Solid Edge part; units mm, degrees
sketch "Sketch1" plane through (0, 0, 0) normal (0, 0, 1) x (1, 0, 0)
  line L0 (12.5075, 35.7826) -> (12.5075, 18.7826)
  line L1 (12.5075, 18.7826) -> (30.5075, 18.7826)
  line L2 (30.5075, 18.7826) -> (46.9075, -0.2273)
  line L3 (46.9075, -0.2273) -> (46.9075, -32.2273)
  line L4 (46.9075, -32.2273) -> (-27.0925, -32.2273)
  line L5 (-27.0925, -32.2273) -> (-27.0925, -0.7273)
  line L6 (-27.0925, -0.7273) -> (-60.0925, -0.7273)
  line L7 (-60.0925, -0.7273) -> (-60.0925, 29.7727)
  line L8 (-60.0925, 29.7727) -> (-27.0925, 29.7727)
  line L9 (-27.0925, 29.7727) -> (12.5075, 35.7826)
  dimension "D1" = 46.9075
  dimension "D2" = 46.9075
  dimension "D3" = 27.0925
  dimension "D4" = 27.0925
  dimension "D5" = 60.0925
  dimension "D6" = 60.0925
  dimension "D7" = 12.5075
  dimension "D8" = 12.5075
extrude "Ajout_matière_1" add sketch "Sketch1" along normal blind 12
sketch "Sketch2" plane through (-11.8425, 1.7776, 12) normal (0, 0, 1) x (1, 0, 0)
  line L0 (-45.25, 24.995) -> (-45.25, 0.495)
  line L1 (-45.25, 0.495) -> (18.1748, 0.495)
  line L2 (44.4511, 0.495) -> (43.1748, 0.495)
  line L3 (39.9995, 14.005) -> (44.4511, 0.495)
  line L4 (21.35, 14.005) -> (39.9995, 14.005)
  line L5 (21.35, 29.6711) -> (21.35, 14.005)
  line L6 (-12.3173, 24.995) -> (21.35, 29.6711)
  line L7 (-45.25, 24.995) -> (-12.3173, 24.995)
  arc A0 (18.1748, 0.495) -> (43.1748, 0.495) centre (30.6748, 0.495) ccw
extrude "Enlèvement_matière_1" cut sketch "Sketch2" against normal blind 11
sketch "Sketch3" plane through (-12.2419, 10.6107, 1) normal (0, 0, 1) x (1, 0, 0)
  circle A0 centre (31.0742, -8.338) radius 1.2899
extrude "Cutout1" cut sketch "Sketch3" along normal through all and the other way through all
sketch "Sketch4" plane through (-11.8425, 1.7776, 0) normal (0, 0, -1) x (0, 1, 0)
  line L0 (-34.005, 58.75) -> (-4.005, 58.75)
  line L1 (-4.005, 58.75) -> (-4.005, -15.25)
  line L2 (-4.005, -15.25) -> (-34.005, -15.25)
  line L3 (-34.005, -15.25) -> (-34.005, 15.75)
  line L4 (-25.505, 15.75) -> (-34.005, 15.75)
  line L5 (-25.505, 26.25) -> (-25.505, 15.75)
  line L6 (-34.005, 26.25) -> (-25.505, 26.25)
  line L7 (-34.005, 26.25) -> (-34.005, 58.75)
  dimension "D1" = 34.005
  dimension "D2" = 25.505
  dimension "D3" = 34.005
extrude "Enlèvement_matière_3" cut sketch "Sketch4" against normal blind 6
sketch "Sketch5" plane through (-6.5925, 1.7776, 12) normal (0, 0, 1) x (0, -1, 0)
  circle A0 centre (28.505, 49) radius 1.5
  circle A1 centre (28.505, 38) radius 1.5
  circle A2 centre (28.505, -5) radius 1.5
  line L0 (24.905, 13) -> (32.105, 13)
  line L1 (32.105, 13) -> (32.105, 6.5)
  line L2 (32.105, 6.5) -> (24.905, 6.5)
  line L3 (24.905, 6.5) -> (24.905, 13)
  dimension "D1" = 28.505
extrude "Cutout2" cut sketch "Sketch5" along normal through all and the other way through all
sketch "Sketch6" plane through (-12.2419, 14.6107, 1) normal (0, 0, 1) x (0, -1, 0)
  circle A0 centre (-8.1719, -6.8505) radius 1.5
  dimension "D1" = 8.1719
extrude "Cutout3" cut sketch "Sketch6" along normal through all and the other way through all
sketch "Sketch7" plane through (-6.5925, 1.7776, 12) normal (0, 0, 1) x (0, -1, 0)
  circle A0 centre (18.005, 46.5) radius 1.5
extrude "Cutout4" cut sketch "Sketch7" along normal through all and the other way through all
sketch "Sketch8" plane through (-6.5925, 1.7776, 12) normal (0, 0, 1) x (-1, 0, 0)
  line L0 (20.5, 2.505) -> (58.2278, 2.505)
  line L1 (58.2278, 2.505) -> (58.2278, -30.8265)
  line L2 (58.2278, -30.8265) -> (20.5, -30.8265)
  line L3 (20.5, -30.8265) -> (20.5, 2.505)
  dimension "D1" = 20.5
  dimension "D2" = 58.2278
extrude "Enlèvement_matière_7" cut sketch "Sketch8" along normal mid plane 65.5466
properties material "Nylon, usage général"
Design review of the part built by this model. Coordinates are the model's own, in mm. A direction names the side the tool comes from. Round coordinates to 2 decimals unless told otherwise and drop trailing zeros. Write each loop counter-clockwise with the first axis right and the second up, starting at its lowest first coordinate (ties: lowest second). Pieces come first, ordered by that corner, then holes. Notation, with made-up numbers: (-4, 80.25) - (33, 80.25) arc R36 cw to (33, 117.25) - close; hole circle Ø2 at (7, 14.5). An arc over 180 degrees is marked (long way). Use a Markdown table: item, result. Add a question column.
1. Clearance check with flat-ended pins moving along their axes: pin 1 (4 mm diameter, centred on x = -19.09, y = 22.78, fed in from +Z); pin 2 (1.8 mm diameter, centred on x = 11.5, z = 3, fed in from +Y); pin 3 (6 mm diameter, centred on y = 20, z = 8.5, fed in from +X); pin 4 (2.5 mm diameter, centred on x = 31.41, y = -26.73, fed in from +Z). State where each tip first meets the part, or that it passes through.
2. We need section A-A (y = -26.5). State the section outline as (x, z) points, then the cut area to 3 significant figures.
3. We need section C-C (z = 4.25). State the section outline as (x, y) points, then the cut area to 3 significant figures.
4. Wall thickness on probe 1 along Y at (x, z) = (2.5, 10.75); probe 2 along Y at (x, z) = (19, 8); probe 3 along Z at (x, y) = (-17.5, -5): over which ranges is each line inside the solid? List them lowest first.
5. We need section B-B (z = 10.75). State the section outline as (x, y) points.
6. For faces 1 (the face through (-26, 26.773, 7)), 2 (the face through (-7.56, 29.08, 6.58)), 3 (the face through (10, -23.727, 3)), list the 3-axis set-ups (+Z, -Z, +X, -X, +Y, -Y) from which the entire face can be reached by the end or side of a thin tool; tool diameter is ignored.
7. We need section D-D (x = -1). State the section outline as (y, z) points.
Output:
| question | item | result |
|---|---|---|
| 1 | pin 1 | stops at z = 1 |
| 1 | pin 2 | stops at y = 35.77 |
| 1 | pin 3 | stops at x = 32.05 |
| 1 | pin 4 | passes through |
| 2 | outline | (-27.09, 6) - (-13.08, 6) - (-13.08, 12) - (-27.09, 12) - close; (-10.11, 6) - (-0.09, 6) - (-0.09, 12) - (-10.11, 12) - close; (6.41, 0) - (14.41, 0) - (14.41, 6) - (29.92, 6) - (29.92, 12) - (6.41, 12) - close; (32.89, 6) - (40.92, 6) - (40.92, 12) - (32.89, 12) - close; (43.89, 6) - (46.91, 6) - (46.91, 12) - (43.89, 12) - close |
| 2 | area | 400 mm2 |
| 3 | outline | (-27.09, -2.23) - (7.17, -2.23) arc R12.5 cw to (6.33, 2.27) - (-27.09, 2.27) - close; (-27.09, 26.77) - (-24.16, 26.77) - (9.51, 31.45) - (9.51, 15.78) - (28.16, 15.78) - (32.61, 2.27) - (31.33, 2.27) arc R12.5 cw to (30.49, -2.23) - (46.91, -2.23) - (46.91, -0.23) - (30.51, 18.78) - (12.51, 18.78) - (12.51, 35.78) - (-27.09, 29.77) - close; (3.91, -32.23) - (14.41, -32.23) - (14.41, -23.73) - (6.41, -23.73) - (6.41, -30.33) - (3.91, -30.33) - close |
| 3 | area | 658 mm2 |
| 4 | probe 1 | y = -32.23 to -30.33, -23.13 to 2.27, 30.48 to 34.26 |
| 4 | probe 2 | y = -32.23 to -10.23, 15.78 to 18.78 |
| 4 | probe 3 | z = 6 to 12 |
| 5 | outline | (-27.09, -32.23) - (46.91, -32.23) - (46.91, -0.23) - (30.51, 18.78) - (12.51, 18.78) - (12.51, 35.78) - (-27.09, 29.77) - (-27.09, 26.77) - (-24.16, 26.77) - (9.51, 31.45) - (9.51, 15.78) - (28.16, 15.78) - (32.61, 2.27) - (31.33, 2.27) arc R12.5 cw to (6.33, 2.27) - (-27.09, 2.27) - close; hole circle Ø3 at (-11.59, -26.73); hole (-0.09, -30.33) - (6.41, -30.33) - (6.41, -23.13) - (-0.09, -23.13) - close; hole circle Ø3 at (31.41, -26.73); hole circle Ø3 at (39.91, -16.23); hole circle Ø3 at (42.41, -26.73) |
| 6 | face 1 | +Z, -X |
| 6 | face 2 | +Z |
| 6 | face 3 | -Z, +X, -X |
| 7 | outline | (-32.23, 6) - (-2.23, 6) - (-2.23, 0) - (33.73, 0) - (33.73, 12) - (29.99, 12) - (29.99, 1) - (2.27, 1) - (2.27, 12) - (-32.23, 12) - close |
